Here's the drawing with two shaded views (mm, measured from the low corner). I have some questions. A direction names the side the tool comes from. Round coordinates to 2 decimals unless told otherwise and drop trailing zeros. Order: outer loops, then holes, each group sorted by start corner. A loop starts at its lowest first (then second) coordinate and runs counter-clockwise, first axis right, second up.
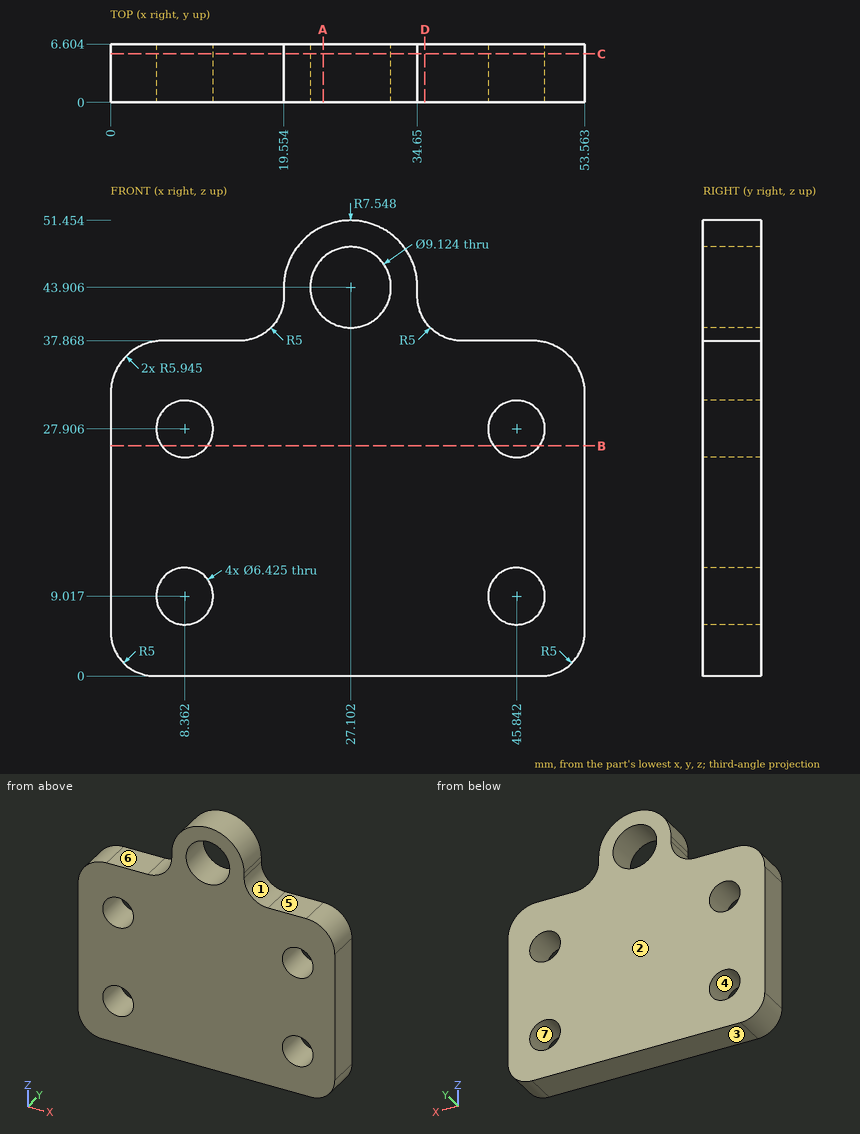
1. I'm going to push flat-ended pins straight in: P1, Ø1.1, axis at y = 2.5, z = 43.5, coming from the +X side; P2, Ø3, axis at y = 2.5, z = 37.5, coming from the -X side. Where does each tip first touch, or does it pass through?
Evaluation:
P1: stops at x = 34.65
P2: stops at x = 1.62
2. If we section it at A-A, the plane x = 24: Write out the boundary of the cut face in (y, z).
Evaluation:
outline: (0, 0) - (6.6, 0) - (6.6, 40.56) - (0, 40.56) - close; (0, 47.25) - (6.6, 47.25) - (6.6, 50.79) - (0, 50.79) - close
3. If we section it at C-C, the plane y = 5.5: State how many separate pieces and enclosed holes the cut face has, and give its area (3 significant figures).
Evaluation:
separate pieces: 1
enclosed holes: 5
area: 2,000 mm2
4. On a 3-axis mill with a long thin cutter (end or side, diameter ignored), from which of +Z, -Z, +X, -X, +Y, -Y can I reach the whole of each face in a straight line? I mean the marked faces 5, 6 and 7. Say none if no direction works.
Evaluation:
face 5: +Z, +X, +Y, -Y
face 6: +Z, -X, +Y, -Y
face 7: +Y, -Y
5. If we section it at B-B, the plane z = 26: Write out the boundary of the cut face in (x, y).
Evaluation:
outline: (0, 0) - (5.78, 0) - (5.78, 6.6) - (0, 6.6) - close; (10.95, 0) - (43.26, 0) - (43.26, 6.6) - (10.95, 6.6) - close; (48.43, 0) - (53.56, 0) - (53.56, 6.6) - (48.43, 6.6) - close
6. If we section it at D-D, the plane x = 35.5: Write out the boundary of the cut face in (y, z).
Evaluation:
outline: (0, 0) - (6.6, 0) - (6.6, 40.08) - (0, 40.08) - close
7. I need wall thicknesses on probe 1 along Z at (x, y) = (43.5, 6.25) (1 decimal); probe 2 along Z at (x, y) = (47, 6); probe 3 along Z at (x, y) = (27, 4.25) (1 decimal). Which ranges of each line are inside material? Lowest first, please.
Evaluation:
probe 1: z = 0 to 6.8, 11.2 to 25.7, 30.1 to 37.9
probe 2: z = 0 to 6.02, 12.01 to 24.91, 30.9 to 37.87
probe 3: z = 0 to 39.3, 48.5 to 51.5
8. If we mould it in two halves opening along Z, with no side actions, what happens to the marked faces 1, 2, 3 and 4? For each: released by +Z, released by -Z, zero draft, split by the parting line, or undercut.
Evaluation:
face 1: released by +Z
face 2: zero draft
face 3: released by -Z
face 4: undercut
